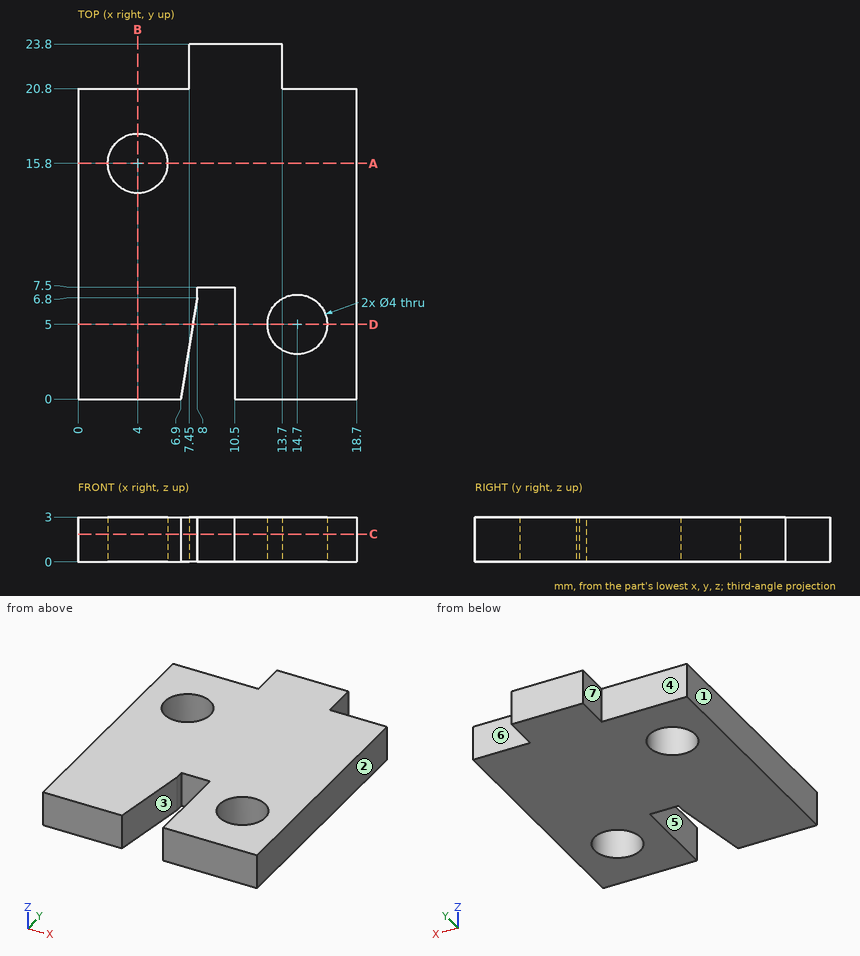
The drawing under review shows one solid part. Ordinate dimensions are in mm from its lowest x, y, z. A direction names the side the tool comes from. Give positions to 0.01 mm unless a question says otherwise; leave off trailing zeros. Write each loop counter-clockwise with the first axis right and the second up, starting at its lowest first coordinate (ties: lowest second). Pieces come first, ordered by that corner, then holes. Notation, with made-up numbers: (28, 53.5) - (43, 53.5) arc R20 cw to (43, 69.5) - close; hole circle Ø11 at (23, 25). An arc over 180 degrees is marked (long way). Answer in a Markdown table with one row per item. Add a question column.
1. We need section B-B on x = 4. Write out the cut boundary in (y, z), then the cut area to 3 significant figures.
2. Draft analysis for pull direction X (two halves, no side actions). For the marked faces 1, 2, 3 and 4, state which applies: +X half, -X half, draft (parallel to the pull), parting line (faces both ways), or undercut.
3. We need section A-A on y = 15.8. Write out the cut boundary in (x, z), then the cut area to 3 significant figures.
4. Tool access review of the marked faces 5, 6 and 7: name each direction out of +Z, -Z, +X, -X, +Y, -Y from which nothing blocks a thin tool from reaching the whole face with its end or side.
5. We need section D-D on y = 5. Write out the cut boundary in (x, z), then the cut area to 3 significant figures.
6. Insertion check: P1, Ø0.9, axis at y = 22.5, z = 1.5, coming from the -X side. The pin has a flat end and moves straight along its axis. Give the tip position at first contact, or say it passes through.
7. We need section C-C on z = 1.85. Write out the cut boundary in (x, y).
8. Wall thickness on line 1 along Y through (x, z) = (4, 1.1); line 2 along Y through (x, z) = (14.7, 0.7); line 3 along Y through (x, z) = (18.25, 1.95): over which ranges is each line inside the solid? List them lowest first. Write a range as [from, to].
Ans:
| question | item | result |
|---|---|---|
| 1 | outline | (0, 0) - (13.8, 0) - (13.8, 3) - (0, 3) - close; (17.8, 0) - (20.8, 0) - (20.8, 3) - (17.8, 3) - close |
| 1 | area | 50.4 mm^2 |
| 2 | face 1 | -X half |
| 2 | face 2 | +X half |
| 2 | face 3 | undercut |
| 2 | face 4 | draft |
| 3 | outline | (0, 0) - (2, 0) - (2, 3) - (0, 3) - close; (6, 0) - (18.7, 0) - (18.7, 3) - (6, 3) - close |
| 3 | area | 44.1 mm^2 |
| 4 | face 5 | +Z, -Z, -Y |
| 4 | face 6 | +Z, -Z, +X, +Y |
| 4 | face 7 | +Z, -Z, -X, +Y |
| 5 | outline | (0, 0) - (7.71, 0) - (7.71, 3) - (0, 3) - close; (10.5, 0) - (12.7, 0) - (12.7, 3) - (10.5, 3) - close; (16.7, 0) - (18.7, 0) - (18.7, 3) - (16.7, 3) - close |
| 5 | area | 35.7 mm^2 |
| 6 | P1 | stops at x = 7.45 |
| 7 | outline | (0, 0) - (6.9, 0) - (8, 6.8) - (8, 7.5) - (10.5, 7.5) - (10.5, 0) - (18.7, 0) - (18.7, 20.8) - (13.7, 20.8) - (13.7, 23.8) - (7.45, 23.8) - (7.45, 20.8) - (0, 20.8) - close; hole circle Ø4 at (4, 15.8); hole circle Ø4 at (14.7, 5) |
| 8 | line 1 | y = [0, 13.8], [17.8, 20.8] |
| 8 | line 2 | y = [0, 3], [7, 20.8] |
| 8 | line 3 | y = [0, 20.8] |
